Autodesk Inventor part; units mm, degrees
ref_plane "Plano inicial" through (0, 0, 0) normal (0, 0, 1) x (1, 0, 0)
ref_plane "Plano final" through (0, 0, 2280) normal (0, 0, 1) x (1, 0, 0)
ref_plane "YZ Plane" through (0, 0, 0) normal (1, 0, 0) x (0, 1, 0)
ref_plane "Plano inicial" through (0, 0, 0) normal (0, 0, 1) x (1, 0, 0)
ref_plane "Plano final" through (0, 0, 2280) normal (0, 0, 1) x (1, 0, 0)
sketch "Rascunho" plane through (0, 0, 0) normal (0, 0, 1) x (1, 0, 0)
  line L0 (-15, -9) -> (-15, 9)
  line L1 (-9, 15) -> (9, 15)
  line L2 (15, 9) -> (15, -9)
  line L3 (9, -15) -> (-9, -15)
  arc A0 (-15, -9) -> (-9, -15) centre (-9, -9) ccw
  arc A1 (15, 9) -> (9, 15) centre (9, 9) ccw
  arc A2 (-9, 15) -> (-15, 9) centre (-9, 9) ccw
  arc A3 (9, -15) -> (15, -9) centre (9, -9) ccw
  arc A4 (-9, 12) -> (-12, 9) centre (-9, 9) ccw
  line L4 (-9, 12) -> (9, 12)
  arc A5 (12, 9) -> (9, 12) centre (9, 9) ccw
  line L5 (12, 9) -> (12, -9)
  arc A6 (9, -12) -> (12, -9) centre (9, -9) ccw
  line L6 (9, -12) -> (-9, -12)
  arc A7 (-12, -9) -> (-9, -12) centre (-9, -9) ccw
  line L7 (-12, -9) -> (-12, 9)
  line L8 (0, 22.7397) -> (0, -22.7397) construction
  line L9 (-22.7397, 0) -> (22.7397, 0) construction
  dimension "d7" = 6
  dimension "d9" = 30
  dimension "d11" = 30
  dimension "d12" = 3
  dimension "d15" = 15
  dimension "d16" = 15
extrude "Corpo" add sketch "Rascunho" along normal up to surface (2280 mm away) from surface at 0
sketch "Sketch3" plane through (0, 0, 0) normal (0, 0, 1) x (1, 0, 0)
  line L0 (0, 0) -> (10, 0)
ref_plane "Work Plane3" through (0, 0, 0) normal (0, -1, 0) x (1, 0, 0)
sketch "Esboço5" plane through (-9, -15, 2280) normal (0, 0, 1) x (1, 0, 0)
  point P0 (9, 15)
sketch "Esboço7" plane through (-15, 9, 0) normal (-1, 0, 0) x (0, 0, 1)
  line L0 (2280, -53.7835) -> (2280, 35.3668)
  circle A0 centre (1840, -9) radius 4
  line L1 (1862, -56.2056) -> (1862, 46.17)
  line L2 (1822, -56.2056) -> (1822, 46.17)
  line L3 (0, -24) -> (2280, -24)
  circle A1 centre (440, -9) radius 4
  line L4 (0, -18) -> (0, 0)
  point P0 (0, -9)
  dimension "d23" = 8
  dimension "d24" = 440
  dimension "d27" = 40
  dimension "d28" = 15
  dimension "d29" = 8
  dimension "d30" = 440
  dimension "d31" = 15
extrude "Extrusão3" cut sketch "Esboço7" against normal through all
sketch "Sketch4" plane through (0, 0, 0) normal (0, -1, 0) x (1, 0, 0)
  line L0 (-2, 0) -> (12, 0)
  line L1 (-2, 2280) -> (12, 2280)
  dimension "d18" = 2280
equation "\"d7\" = G_IR"
equation "\"d9\" = G_W"
equation "\"d11\" = G_H"
equation "\"d12\" = G_T"
equation "\"d15\" = 0.5 * d9"
equation "\"d16\" = 0.5 * d11"
equation "\"d3\" = G_L"
equation "\"G_W\" = 30"
equation "\"G_H\" = 30"
equation "\"G_T\" = 3"
equation "\"G_IR\" = 6"
equation "\"G_L\" = d18"
equation "\"G_OFFSET_START\" = 0"
equation "\"G_OFFSET_END\" = 0"
properties part number "Perfil tubo - 30x30x3 - 2280" material "Aço, suave"
Model file for the job. Use its own axes, mm. Give positions to 0.01 mm unless a question says otherwise; leave off trailing zeros. Loops run counter-clockwise (first coordinate to the right, second up) from the corner with the lowest first, then second, coordinate; pieces in that order, holes last. Notation, with made-up numbers: (41, 61.25) - (92, 61.25) arc R10 ccw to (92, 73.25) - close; hole circle Ø3 at (38.25, -17.75). An arc over 180 degrees is marked (long way). One line per item, written item: value. Start each with the question number.
1. Slice it at A-A (x = 3.75). List the corners of the cut face in (y, z).
2. Probe L1, parallel to Y at x = -8.5, z = 386; L2, parallel to Y at x = -14.25, z = 440. List the from-to ranges inside material, lowest first. Write a range as from..to.
3. Slice it at B-B (z = 976.5). List the corners of the cut face in (x, y), plus the area to 3 significant figures.
Solution:
1. outline: (-15, 0) - (-12, 0) - (-12, 2280) - (-15, 2280) - close; (12, 0) - (15, 0) - (15, 2280) - (12, 2280) - close
2. L1: y = -15..-12, 12..15
2. L2: y = -11.9..-4, 4..11.9
3. outline: (-15, -9) arc R6 ccw to (-9, -15) - (9, -15) arc R6 ccw to (15, -9) - (15, 9) arc R6 ccw to (9, 15) - (-9, 15) arc R6 ccw to (-15, 9) - close; hole (-12, -9) arc R3 ccw to (-9, -12) - (9, -12) arc R3 ccw to (12, -9) - (12, 9) arc R3 ccw to (9, 12) - (-9, 12) arc R3 ccw to (-12, 9) - close
3. area: 301 mm^2
